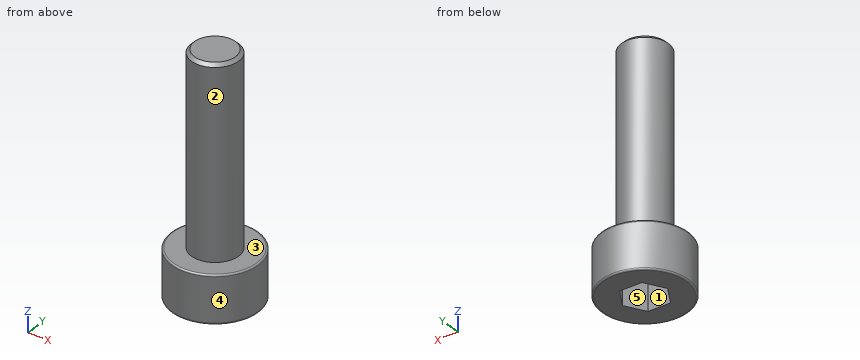
Autodesk Inventor part; units mm, degrees
ref_plane "YZ Plane" through (0, 0, 0) normal (1, 0, 0) x (0, 1, 0)
ref_plane "XZ Plane" through (0, 0, 0) normal (0, 1, 0) x (-1, 0, 0)
ref_plane "XY Plane" through (0, 0, 0) normal (0, 0, 1) x (1, 0, 0)
sketch "Sketch1" plane through (0, 0, 0) normal (0, 0, 1) x (1, 0, 0)
  circle A0 centre (0, 0) radius 2.75
extrude "Extrusion3" add sketch "Sketch1" against normal blind 3
sketch "Sketch2" plane through (0, 0, 0) normal (0, 0, 1) x (1, 0, 0)
  circle A0 centre (0, 0) radius 1.5
extrude "Extrusion2" add sketch "Sketch2" along normal blind 12
sketch "Sketch3" plane through (0, 0, -3) normal (0, 0, -1) x (-1, 0, 0)
  line L0 (-0.7217, 1.25) -> (-1.4434, 0)
  line L1 (0.7217, -1.25) -> (1.4434, 0)
  line L2 (1.4434, 0) -> (0.7217, 1.25)
  line L3 (-1.4434, 0) -> (-0.7217, -1.25)
  line L4 (0.7217, 1.25) -> (-0.7217, 1.25)
  line L5 (-0.7217, -1.25) -> (0.7217, -1.25)
extrude "Extrusion1" cut sketch "Sketch3" against normal blind 3
fillet "Fillet2" radius 0.1 1 edges at (-2.75, 0, -3)
fillet "Fillet1" radius 0.1 1 edges at (-2.75, 0, 0)
chamfer "Chamfer1" distance 0.2 angle 45 1 edges at (-1.5, 0, 12)
properties part number "DIN 912 M3 12 mm"
Source: CAD feature listing. Evaluate the final solid. Frame: model axes, mm. Face numbers are marked on the shaded views. A direction names the side the tool comes from. Round coordinates to 2 decimals unless told otherwise and drop trailing zeros. Loops run counter-clockwise (first coordinate to the right, second up) from the corner with the lowest first, then second, coordinate; pieces in that order, holes last. Notation, with made-up numbers: (-24, 24.25) - (-2, 24.25) arc R18 cw to (-2, 49.25) - close; hole circle Ø3 at (22, 79). An arc over 180 degrees is marked (long way). Use CSV: the item, a comma, the result in double quotes.
Q1. Section query B-B, the plane z = 1.75. Output: boundary loops of the cut face in (x, y).
Reported:
outline,"circle Ø3 at (0, 0)"
Q2. Pin query (flat end, axial travel): pin 1 Ø1 at (y, z) = (-1.5, 6.5) entering from +X; pin 2 Ø1.5 at (y, z) = (0.5, 1) entering from -X. Return the tip coordinate at first contact, or that it passes through.
Reported:
pin 1,"x = 1.12"
pin 2,"x = -1.5"
Q3. Ray query, line 1 along X through (y, z) = (-0.1, 9.25); line 2 along Z through (x, y) = (1.95, 0.7); line 3 along Z through (x, y) = (-0.05, -0.55). Return the intervals inside material, ascending.
Reported:
line 1,"-1.5 to 1.5"
line 2,"-3 to 0"
line 3,"0 to 12"
Q4. Section query A-A, the plane x = 0. Output: boundary loops of the cut face in (y, z).
Reported:
outline,"(-2.75, -2.9) arc R0.1 ccw to (-2.65, -3) - (-1.25, -3) - (-1.25, 0) - (1.25, 0) - (1.25, -3) - (2.65, -3) arc R0.1 ccw to (2.75, -2.9) - (2.75, -0.1) arc R0.1 ccw to (2.65, 0) - (1.5, 0) - (1.5, 11.8) - (1.3, 12) - (-1.3, 12) - (-1.5, 11.8) - (-1.5, 0) - (-2.65, 0) arc R0.1 ccw to (-2.75, -0.1) - close"
Q5. Mould query, pull axis Y, two halves, no side actions, for the marked faces 1, 2 and 3. Classes: pulls with the +Y half, pulls with the -Y half, needs draft (parallel to the pull), parting line crosses it, or undercut.
Reported:
face 1,"undercut"
face 2,"parting line crosses it"
face 3,"needs draft"
Q6. Reachability of the marked faces 4 and 5 from +Z, -Z, +X, -X, +Y, -Y: full face, straight path, thin tool, end or side. Return the list, or none.
Reported:
face 4,"+Z, -Z"
face 5,"-Z"
